Verification items for the finished model (mm, model axes). A direction names the side the tool comes from. Give positions to 0.01 mm unless a question says otherwise; leave off trailing zeros. Order: outer loops, then holes, each group sorted by start corner. A loop starts at its lowest first (then second) coordinate and runs counter-clockwise, first axis right, second up.
(1) Scan lines: L1, parallel to Z at x = 1, y = 0.75; L2, parallel to Y at x = 0.75, z = -4; L3, parallel to Y at x = 1.25, z = -4.75. Record each from-to range of solid material in increasing order.
(2) Access from +Z, -Z, +X, -X, +Y, -Y to the whole of each face (thin tool, end or side, straight path). Record for faces 1 (the face through (0, 2, -1)), 2 (the face through (0.63, 1.08, 6.27)), 3 (the face through (0, 0, -7.5)).
(3) Gauge pin test, flat ends, axial feed: pin 1 (4 mm diameter, centred on y = -0.5, z = 3, fed in from +X); pin 2 (0.7 mm diameter, centred on y = 0.5, z = 6, fed in from +X). Record the tip position at first contact, or that the pin passes through.
(4) Sectioned sample at A-A on y = 0. Record the cut outline in (x, z), plus the area to 3 significant figures.
(5) Mould release check, pull along Y, two halves, no side actions. Record for faces 4 (the face through (2, 0, 7.5)), 5 (the face through (0.867, 3.905, 7.196)), 6 (the face through (-0.63, -1.08, 6.27)): pulls with the +Y half, pulls with the -Y half, needs draft (parallel to the pull), parting line crosses it, or undercut.
(6) Sectioned sample at B-B on z = 1. Record the cut outline in (x, y).
```python
from build123d import *

# Parameters (mm, degrees)
CHAMFER_1_SIZE      = 0.5
CUT_EXTRUDE_1_DEPTH = 2.5


with BuildPart() as part:
    # 草图1 → 旋转1 (revolve)
    with BuildSketch(Plane(origin=(0, 0, 0), x_dir=(0, 0, -1), z_dir=(1, 0, 0)), mode=Mode.PRIVATE) as revolve_1_sk:
        Polygon((-7.5, 0), (-7.5, 4), (-6.9, 4), (-4.9, 2), (7.5, 2), (7.5, 0), align=None)
    revolve(revolve_1_sk.sketch.rotate(Axis((0, 0, -7.5), (0, 0, 1)), 90), axis=Axis((0, 0, -7.5), (0, 0, 1)))

    # 倒角1
    chamfer_1_edges = [part.edges().sort_by_distance(p)[0] for p in [
        (2, 0, -7.5),
    ]]
    chamfer(chamfer_1_edges, length=CHAMFER_1_SIZE)

    # 草图2 → 切除-拉伸1 (cut)
    with BuildSketch(Plane.XY.offset(7.5)):
        Polygon((0, 1.443375673), (-1.25, 0.721687836), (-1.25, -0.721687836), (0, -1.443375673), (1.25, -0.721687836), (1.25, 0.721687836), align=None)
    extrude(amount=-CUT_EXTRUDE_1_DEPTH, mode=Mode.SUBTRACT)


solid = part.part
```
Ans:
1. L1: z = -7.5 to 5
1. L2: y = -1.85 to 1.85
1. L3: y = -1.56 to 1.56
2. face 1: -Z
2. face 2: +Z
2. face 3: -Z, +X, -X, +Y, -Y
3. pin 1: stops at x = 2.07
3. pin 2: stops at x = 3.42
4. outline: (-4, 6.9) - (-2, 4.9) - (-2, -7) - (-1.5, -7.5) - (1.5, -7.5) - (2, -7) - (2, 4.9) - (4, 6.9) - (4, 7.5) - (1.25, 7.5) - (1.25, 5) - (-1.25, 5) - (-1.25, 7.5) - (-4, 7.5) - close
4. area: 59.9 mm2
5. face 4: needs draft
5. face 5: parting line crosses it
5. face 6: undercut
6. outline: circle Ø4 at (0, 0)
